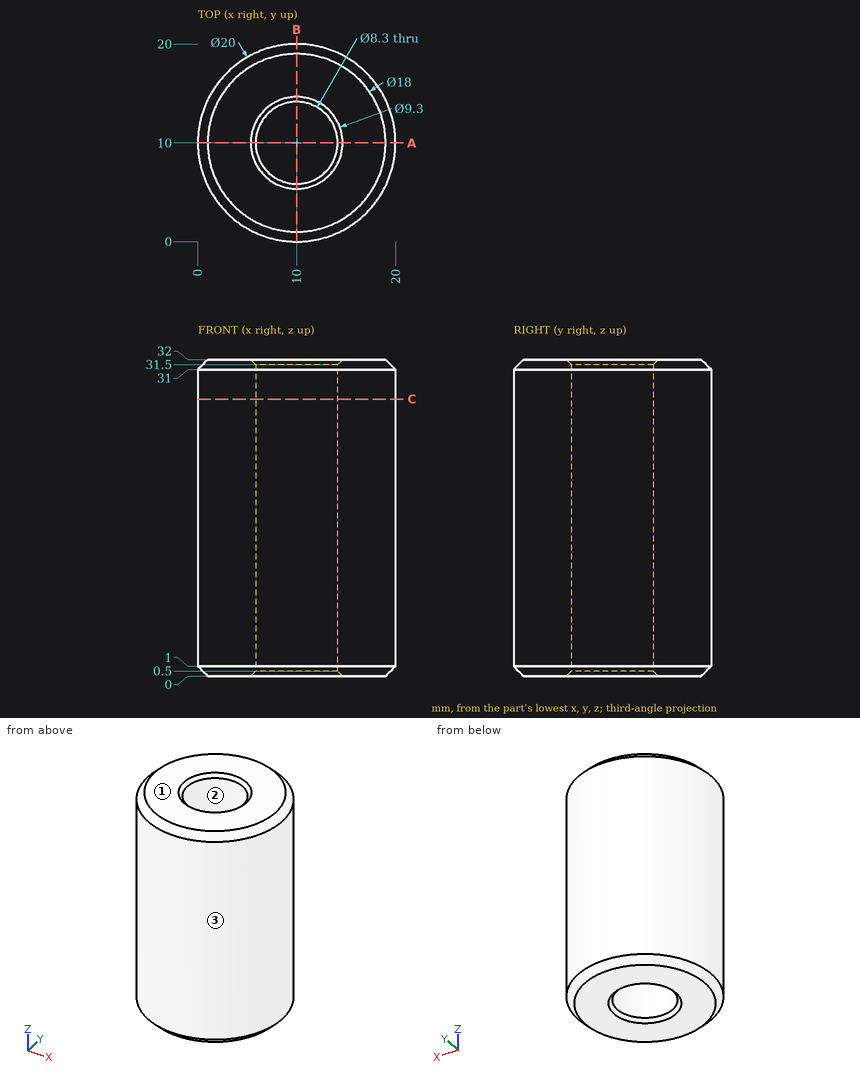
For this review, use the dimensioned drawing (mm, ordinates from the lowest corner) and the shaded views. Round coordinates to 2 decimals unless told otherwise and drop trailing zeros. Loops run counter-clockwise (first coordinate to the right, second up) from the corner with the lowest first, then second, coordinate; pieces in that order, holes last. Notation, with made-up numbers: M -37,60.5 L 20,60.5 A16 cw 20,86.5 Z; hole C -25,59.5 d6. An arc over 180 degrees is marked long. Answer as a JSON object with one key per item and string values.
(1) To check wall thickness, follow line 1 along Y through (x, z) = (10, 18.5); line 2 along X through (y, z) = (13.5, 12.5); line 3 along Y through (x, z) = (7, 16). State the ranges of each line that lie inside material, in increasing order.
Resolved:
{"line 1": "0 to 5.85, 14.15 to 20", "line 2": "0.63 to 7.77, 12.23 to 19.37", "line 3": "0.46 to 7.13, 12.87 to 19.54"}
(2) Take a section at A-A on y = 10. Give the boundary of the cut face in (x, z).
Resolved:
{"outline": "M 0,1 L 1,0 L 5.35,0 L 5.85,0.5 L 5.85,31.5 L 5.35,32 L 1,32 L 0,31 Z; M 14.15,0.5 L 14.65,0 L 19,0 L 20,1 L 20,31 L 19,32 L 14.65,32 L 14.15,31.5 Z"}
(3) Take a section at C-C on z = 28. Give the boundary of the cut face in (x, y), and give its area (3 significant figures).
Resolved:
{"outline": "C 10,10 d20; hole C 10,10 d8.3", "area": "260 mm²"}
(4) Draft analysis for pull direction X (two halves, no side actions). For the marked faces 1, 2 and 3, state which applies: released by +X, released by -X, zero draft, split by the parting line, or undercut.
Resolved:
{"face 1": "zero draft", "face 2": "undercut", "face 3": "split by the parting line"}
(5) Clearance check with flat-ended pins moving along their axes: P1, Ø1.5, axis at x = 3.5, z = 15.5, coming from the -Y side; P2, Ø8, axis at y = 2.5, z = 26.5, coming from the -X side; P3, Ø1.5, axis at y = 17, z = 11, coming from the +X side. State where each tip first meets the part, or that it passes through.
Resolved:
{"P1": "y = 1.82", "P2": "x = 0.63", "P3": "x = 17.81"}
